Geometry: see drawing. Coordinates: mm, zero at the bounding-box minimum. A direction names the side the tool comes from. Round coordinates to 2 decimals unless told otherwise and drop trailing zeros. Loops run counter-clockwise (first coordinate to the right, second up) from the corner with the lowest first, then second, coordinate; pieces in that order, holes last. Notation, with made-up numbers: (49.25, 28) -> (84.25, 28) arc R14 ccw to (84.25, 55) -> close; hole circle Ø2 at (74, -38). An arc over 180 degrees is marked (long way). Write item = value, one per line.
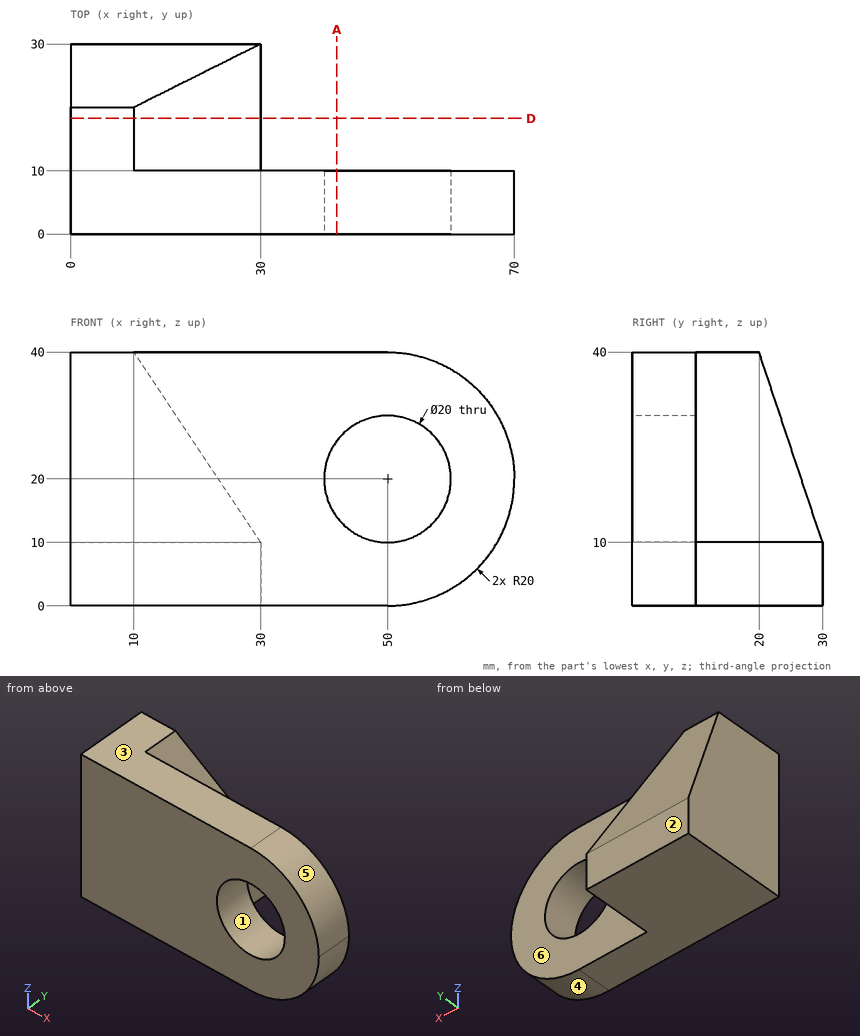
1. Section query D-D (y = 18.25). Return the cut outline in (x, z).
Evaluation:
outline = (0, 0) -> (30, 0) -> (30, 10) -> (10, 40) -> (0, 40) -> close
2. Mould query, pull axis Z, two halves, no side actions, for the marked faces 1, 2, 3 and 4. Classes: released by +Z, released by -Z, zero draft, split by the parting line, or undercut.
Evaluation:
face_1 = undercut
face_2 = zero draft
face_3 = released by +Z
face_4 = released by -Z
3. Line query: probe 1 along Z at (x, y) = (50, 2.5); probe 2 along X at (y, z) = (5, 20); probe 3 along X at (y, z) = (15.75, 8.5). Output: solid intervals per line, ascending. Write a range as from..to.
Evaluation:
probe_1 = 0..10, 30..40
probe_2 = 0..40, 60..70
probe_3 = 0..30
4. Set-up query: the marked faces 5 and 6. Return all of +Z, -Z, +X, -X, +Y, -Y with unobstructed straight access to the full face (end or side cutting, diameter ignored); none if empty.
Evaluation:
face_5 = +Z, +X, +Y, -Y
face_6 = +Z, +X, +Y
5. Section query A-A (x = 42). Return the cut outline in (y, z).
Evaluation:
outline = (0, 0) -> (10, 0) -> (10, 14) -> (0, 14) -> close; (0, 26) -> (10, 26) -> (10, 40) -> (0, 40) -> close
6. Contact query for flat-ended pins moving along their axis: pin 1 Ø5 at (y, z) = (19.5, 5) entering from +X; pin 2 Ø12 at (x, z) = (44, 25) entering from +Y; pin 3 Ø8 at (x, z) = (51.5, 22.5) entering from +Y; pin 4 Ø1.5 at (x, y) = (26.5, 19) entering from +Z (1 decimal). Output: stop coordinate, or through.
Evaluation:
pin_1 = 30
pin_2 = 10
pin_3 = through
pin_4 = 16.4
